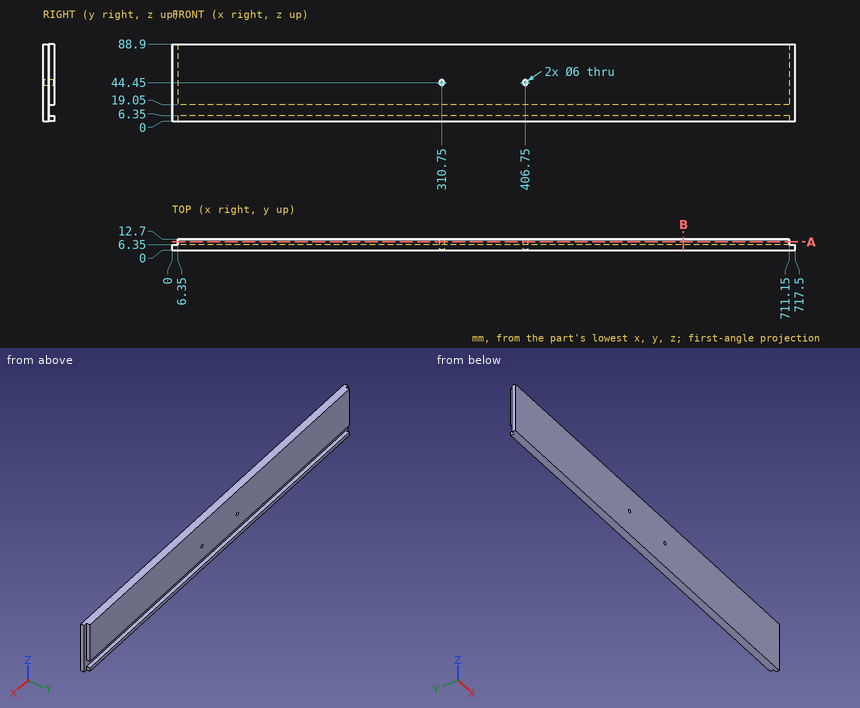
Check sheet for the drawn part. Datum: minimum x, y, z corner. Units: mm. Coordinates: 2 decimals unless noted, no trailing zeros. Order: outer loops, then holes, each group sorted by start corner. A loop starts at its lowest first (then second) coordinate and runs counter-clockwise, first axis right, second up. Notation, with made-up numbers: M 72.5,35.25 L 82.5,35.25 A29 ccw 82.5,73.25 Z; hole C 21,-2 d4. An arc over 180 degrees is marked long. One line per item, written item: value. Start each with the question number.
Item 1: Scan lines: probe 1 along X at (y, z) = (9.25, 44.45); probe 2 along X at (y, z) = (6, 44.45); probe 3 along Z at (x, y) = (612, 10.75). Record each from-to range of solid material in increasing order.
Item 2: Sectioned sample at A-A (y = 9.5). Enter the section's corners in (x, z).
Item 3: Sectioned sample at B-B (x = 589). Enter the section's corners in (y, z), then the cut area to 3 significant figures.
Item 4: Gauge pin test, flat ends, axial feed: pin 1 (6 mm diameter, centred on y = 3, z = 50.5, fed in from -X); pin 2 (3 mm diameter, centred on y = 8.5, z = 69.5, fed in from +X); pin 3 (4 mm diameter, centred on x = 101.5, z = 9.5, fed in from +Y). Record the tip position at first contact, or that the pin passes through.
Conclusion:
1. probe 1: x = 6.35 to 307.75, 313.75 to 403.75, 409.75 to 711.15
1. probe 2: x = 0 to 307.75, 313.75 to 403.75, 409.75 to 717.5
1. probe 3: z = 0 to 6.35, 19.05 to 88.9
2. outline: M 6.35,0 L 711.15,0 L 711.15,6.35 L 6.35,6.35 Z; M 6.35,19.05 L 711.15,19.05 L 711.15,88.9 L 6.35,88.9 Z; hole C 310.75,44.45 d6; hole C 406.75,44.45 d6
3. outline: M 0,0 L 12.7,0 L 12.7,6.35 L 6.35,6.35 L 6.35,19.05 L 12.7,19.05 L 12.7,88.9 L 0,88.9 Z
3. area: 1,050 mm^2
4. pin 1: stops at x = 0
4. pin 2: stops at x = 711.15
4. pin 3: stops at y = 6.35
